Here's the drawing with two shaded views (mm, measured from the low corner). I have some questions. Round coordinates to 2 decimals unless told otherwise and drop trailing zeros. Order: outer loops, then holes, each group sorted by start corner. A loop starts at its lowest first (then second) coordinate and runs counter-clockwise, first axis right, second up.
Q1. If we section it at A-A (z = 11): Please give me the cut outline in (x, y).
Q2. If we section it at D-D (z = 6.25): Please give me the cut outline in (x, y), plus the area to 3 significant figures.
Q3. Will these pins go through, and if not, where does the flat tip stop? P1, Ø0.8, axis at y = 2, z = 7, coming from the +X side; P2, Ø3, axis at x = 14, z = 10, coming from the +Y side; P3, Ø2.5, axis at x = 3, z = 11, coming from the -Y side.
Q4. If we section it at B-B (x = 3): Please give me the cut outline in (y, z).
Q5. If we section it at C-C (x = 6.5): Please give me the cut outline in (y, z), plus the area to 3 significant figures.
Q6. If I drill on line 1 (X direction, y = 0.95, z = 11); line 2 (Y direction, x = 12.5, z = 3.25); line 3 (X direction, y = 1.6, z = 5), over which ranges is the centre line in solid material (lowest first)?
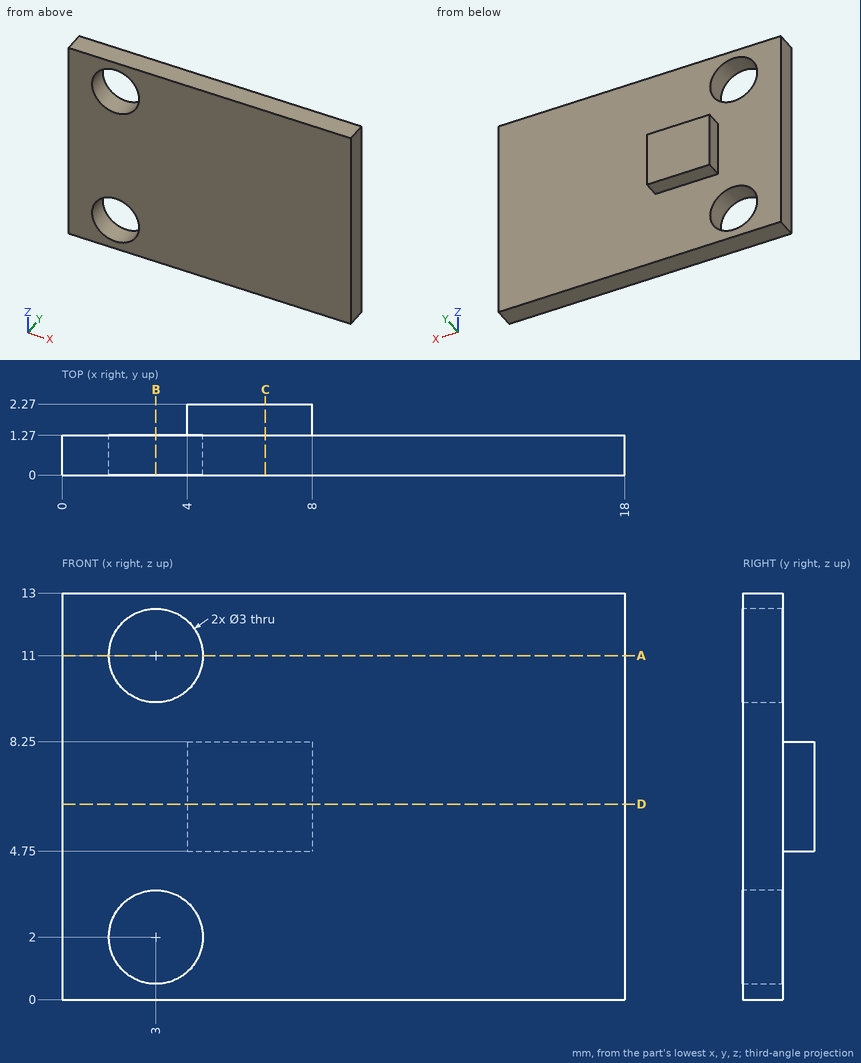
Solution:
1. outline: (0, 0) - (1.5, 0) - (1.5, 1.27) - (0, 1.27) - close; (4.5, 0) - (18, 0) - (18, 1.27) - (4.5, 1.27) - close
2. outline: (0, 0) - (18, 0) - (18, 1.27) - (8, 1.27) - (8, 2.27) - (4, 2.27) - (4, 1.27) - (0, 1.27) - close
2. area: 26.9 mm2
3. P1: stops at x = 8
3. P2: stops at y = 1.27
3. P3: passes through
4. outline: (0, 0) - (1.27, 0) - (1.27, 0.5) - (0, 0.5) - close; (0, 3.5) - (1.27, 3.5) - (1.27, 9.5) - (0, 9.5) - close; (0, 12.5) - (1.27, 12.5) - (1.27, 13) - (0, 13) - close
5. outline: (0, 0) - (1.27, 0) - (1.27, 4.75) - (2.27, 4.75) - (2.27, 8.25) - (1.27, 8.25) - (1.27, 13) - (0, 13) - close
5. area: 20.0 mm2
6. line 1: x = 0 to 1.5, 4.5 to 18
6. line 2: y = 0 to 1.27
6. line 3: x = 4 to 8
